```python
from build123d import *

# Parameters (mm, degrees)
SKETCH_1_W                  = 31
SKETCH_1_H                  = 37
EXTRUDE_1_DEPTH             = 30
HOLE_WIZARD_M4_1_AT_2_COUNT = 2
HOLE_WIZARD_M4_1_AT_2_PITCH = 15
HOLE_WIZARD_M4_1_AT_3_COUNT = 2
HOLE_WIZARD_M4_1_AT_3_PITCH = 23.430749028
HOLE_WIZARD_M4_1_AT_4_COUNT = 2
HOLE_WIZARD_M4_1_AT_4_PITCH = 18
HOLE_WIZARD_M4_2_D          = 3.3
HOLE_WIZARD_M4_2_DEPTH      = 10
HOLE_WIZARD_M4_2_TIP        = 0.991420021
SKETCH_8_R                  = 9.5
CUT_EXTRUDE_1_DEPTH         = 9.7
SKETCH_9_R                  = 8.65
CUT_EXTRUDE_2_DEPTH         = 3.3
FILLET_1_R                  = 2
CHAMFER_1_SIZE              = 1


with BuildPart() as part:
    # 草图1 → 凸台-拉伸1 (new body)
    with BuildSketch(Plane.XY):
        Rectangle(SKETCH_1_W, SKETCH_1_H)
    extrude(amount=EXTRUDE_1_DEPTH)

    # 草图4 → M4 螺纹孔1 (revolve, cut)
    with BuildSketch(Plane(origin=(-7.5, 18.5, 6), x_dir=(0, 0, 1), z_dir=(1, 0, 0))):
        Polygon((0, 0), (0, 9.991420021), (1.65, 9), (1.65, 0), align=None)
    hole_wizard_m4_1 = revolve(axis=Axis((-7.5, 24.85, 6), (0, -1, 0)), mode=Mode.SUBTRACT)

    # M4 螺纹孔1 at 2: M4 螺纹孔1 ×2
    with Locations(*[(i * HOLE_WIZARD_M4_1_AT_2_PITCH, 0, 0) for i in range(1, HOLE_WIZARD_M4_1_AT_2_COUNT)]):
        add(hole_wizard_m4_1, mode=Mode.SUBTRACT)

    # M4 螺纹孔1 at 3: M4 螺纹孔1 ×2
    with Locations(*[Vector(0.6401843996644799, 0, 0.7682212795973757) * (i * HOLE_WIZARD_M4_1_AT_3_PITCH) for i in range(1, HOLE_WIZARD_M4_1_AT_3_COUNT)]):
        add(hole_wizard_m4_1, mode=Mode.SUBTRACT)

    # M4 螺纹孔1 at 4: M4 螺纹孔1 ×2
    with Locations(*[(0, 0, i * HOLE_WIZARD_M4_1_AT_4_PITCH) for i in range(1, HOLE_WIZARD_M4_1_AT_4_COUNT)]):
        add(hole_wizard_m4_1, mode=Mode.SUBTRACT)

    # 镜向1: M4 螺纹孔1 across plane
    add(hole_wizard_m4_1.mirror(Plane.ZX), mode=Mode.SUBTRACT)

    # 镜向1 copy 1 sketch → 镜向1 copy 1 (revolve, cut)
    with BuildSketch(Plane(origin=(7.5, -18.5, 6), x_dir=(0, 0, 1), z_dir=(1, 0, 0))):
        Polygon((0, 0), (0, -9.991420021), (1.65, -9), (1.65, 0), align=None)
    revolve(axis=Axis((7.5, -24.85, 6), (0, -1, 0)), mode=Mode.SUBTRACT)

    # 镜向1 copy 2 sketch → 镜向1 copy 2 (revolve, cut)
    with BuildSketch(Plane(origin=(7.5, -18.5, 24), x_dir=(0, 0, 1), z_dir=(1, 0, 0))):
        Polygon((0, 0), (0, -9.991420021), (1.65, -9), (1.65, 0), align=None)
    revolve(axis=Axis((7.5, -24.85, 24), (0, -1, 0)), mode=Mode.SUBTRACT)

    # 镜向1 copy 3 sketch → 镜向1 copy 3 (revolve, cut)
    with BuildSketch(Plane(origin=(-7.5, -18.5, 24), x_dir=(0, 0, 1), z_dir=(1, 0, 0))):
        Polygon((0, 0), (0, -9.991420021), (1.65, -9), (1.65, 0), align=None)
    revolve(axis=Axis((-7.5, -24.85, 24), (0, -1, 0)), mode=Mode.SUBTRACT)

    # M4 螺纹孔2
    with Locations(Plane.ZY.offset(15.5)):
        with Locations((11, 12.5), (19, 12.5), (19, -12.5), (11, -12.5)):
            Hole(HOLE_WIZARD_M4_2_D / 2, depth=HOLE_WIZARD_M4_2_DEPTH)
            with Locations((0, 0, -(HOLE_WIZARD_M4_2_DEPTH + HOLE_WIZARD_M4_2_TIP / 2))):  # 118° drill point
                Cone(0, HOLE_WIZARD_M4_2_D / 2, HOLE_WIZARD_M4_2_TIP, mode=Mode.SUBTRACT)

    # 草图8 → 切除-拉伸1 (cut)
    with BuildSketch(Plane(origin=(0, 0, 0), x_dir=(-1, 0, 0), z_dir=(0, 0, -1))):
        Circle(SKETCH_8_R)
    extrude(amount=-CUT_EXTRUDE_1_DEPTH, mode=Mode.SUBTRACT)

    # 草图9 → 切除-拉伸2 (cut)
    with BuildSketch(Plane(origin=(0, 0, 9.7), x_dir=(-1, 0, 0), z_dir=(0, 0, -1))):
        Circle(SKETCH_9_R)
    extrude(amount=-CUT_EXTRUDE_2_DEPTH, mode=Mode.SUBTRACT)

    # 圆角1
    fillet_1_edges = [part.edges().sort_by_distance(p)[0] for p in [
        (15.5, -18.5, 15),
        (-15.5, -18.5, 15),
        (-15.5, 18.5, 15),
        (15.5, 18.5, 15),
    ]]
    fillet(fillet_1_edges, radius=FILLET_1_R)

    # 倒角1
    chamfer_1_edges = [part.edges().sort_by_distance(p)[0] for p in [
        (9.5, 0, 0),
    ]]
    chamfer(chamfer_1_edges, length=CHAMFER_1_SIZE)


solid = part.part
```
Model file for the job. Use its own axes, mm. A direction names the side the tool comes from. Coordinates: 2 decimals unless noted, no trailing zeros. Loops run counter-clockwise (first coordinate to the right, second up) from the corner with the lowest first, then second, coordinate; pieces in that order, holes last. Notation, with made-up numbers: (37, 6.25) - (60, 6.25) arc R9 ccw to (60, 15.25) - close; hole circle Ø4 at (87.25, -20.5). An arc over 180 degrees is marked (long way). Answer as a JSON object with one key per item and string values. Group by question number.
(1) Flat gauge pins, fed straight in: pin 1 (5.5 mm diameter, centred on x = 7.5, z = 6, fed in from +Y); pin 2 (3 mm diameter, centred on x = 7.5, z = 24, fed in from +Y); pin 3 (5 mm diameter, centred on x = 3.5, y = 3.5, fed in from -Z); pin 4 (3 mm diameter, centred on x = 7.5, z = 24, fed in from -Y). Where does each tip first touch, or does it go through?
(2) Cut at D-D (x = 0). Give the cut face in (y, z), then the cut area to 3 significant figures.
(3) Cut at C-C (z = 2.5). Give the cut face in (x, y).
(4) Probe line 1 along Y through (x, z) = (-10.25, 19); line 2 along Z through (x, y) = (7.5, -13.5); line 3 along X through (y, z) = (16.25, 6). List the from-to ranges inside material, lowest first.
(5) Tool access for faces 1 (the face through (-4.38, -8.43, 5.29)), 2 (the face through (-7.57, 14.06, 4.35)), 3 (the face through (0, 18.5, 15)), 4 (the face through (7.43, -14.06, 4.35)): list every direction of +Z, -Z, +X, -X, +Y, -Y with a clear straight run to the whole face (end or side of a thin tool).
(6) Two-plate mould, pull along Y, no slides. Class faces 5 (the face through (7.6, -8.7, 24.3)), 6 (the face through (-7.57, -14.06, 22.35)), 7 (the face through (-8.25, 2.6, 11.33)): released by +Y, released by -Y, zero draft, split by the parting line, or undercut.
(7) Cut at B-B (y = 0). Give the cut face in (x, z), then the cut area to 3 significant figures.
(8) Cut at A-A (x = -12). Give the cut face in (y, z).
Geometry says:
{
 "1": {"pin 1": "stops at y = 18.5", "pin 2": "stops at y = 9.41", "pin 3": "stops at z = 13", "pin 4": "stops at y = -9.41"},
 "2": {"outline": "(-18.5, 0) - (-10.5, 0) - (-9.5, 1) - (-9.5, 9.7) - (-8.65, 9.7) - (-8.65, 13) - (8.65, 13) - (8.65, 9.7) - (9.5, 9.7) - (9.5, 1) - (10.5, 0) - (18.5, 0) - (18.5, 30) - (-18.5, 30) - close", "area": "868 mm^2"},
 "3": {"outline": "(-15.5, -16.5) arc R2 ccw to (-13.5, -18.5) - (13.5, -18.5) arc R2 ccw to (15.5, -16.5) - (15.5, 16.5) arc R2 ccw to (13.5, 18.5) - (-13.5, 18.5) arc R2 ccw to (-15.5, 16.5) - close; hole circle Ø19 at (0, 0)"},
 "4": {"line 1": "y = -18.5 to -14.15, -10.85 to 10.85, 14.15 to 18.5", "line 2": "z = 0 to 4.35, 7.65 to 22.35, 25.65 to 30", "line 3": "x = -15.5 to -9.15, -5.85 to 5.85, 9.15 to 15.5"},
 "5": {"face 1": "-Z", "face 2": "+Y", "face 3": "+Z, -Z, +X, -X, +Y", "face 4": "-Y"},
 "6": {"face 5": "released by -Y", "face 6": "zero draft", "face 7": "undercut"},
 "7": {"outline": "(-15.5, 0) - (-10.5, 0) - (-9.5, 1) - (-9.5, 9.7) - (-8.65, 9.7) - (-8.65, 13) - (8.65, 13) - (8.65, 9.7) - (9.5, 9.7) - (9.5, 1) - (10.5, 0) - (15.5, 0) - (15.5, 30) - (-15.5, 30) - close", "area": "688 mm^2"},
 "8": {"outline": "(-18.5, 0) - (18.5, 0) - (18.5, 30) - (-18.5, 30) - close; hole circle Ø3.3 at (-12.5, 11); hole circle Ø3.3 at (-12.5, 19); hole circle Ø3.3 at (12.5, 11); hole circle Ø3.3 at (12.5, 19)"}
}
